```python
from build123d import *

# Parameters (mm, degrees)
SKETCH1_W           = 40.64
SKETCH1_H           = 32
BOSS_EXTRUDE1_DEPTH = 4
SKETCH2_R           = 8
BOSS_EXTRUDE2_DEPTH = 3.6
SKETCH3_W           = 3.3
SKETCH3_H           = 32
BOSS_EXTRUDE3_DEPTH = 3.6
FILLET1_R           = 0.5


with BuildPart() as part:
    # Sketch1 → Boss-Extrude1 (new body)
    with BuildSketch(Plane(origin=(0, 0, 0), x_dir=(1, 0, 0), z_dir=(0, 1, 0))):
        Rectangle(SKETCH1_W, SKETCH1_H)
    extrude(amount=BOSS_EXTRUDE1_DEPTH)

    # Sketch2 → Boss-Extrude2 (add)
    with BuildSketch(Plane(origin=(0, 4, 0), x_dir=(1, 0, 0), z_dir=(0, 1, 0))):
        with Locations(Location((0, 0, 0), (0, 0, 270))):
            Circle(SKETCH2_R)
    extrude(amount=BOSS_EXTRUDE2_DEPTH)

    # Sketch3 → Boss-Extrude3 (add)
    with BuildSketch(Plane(origin=(0, 4, 0), x_dir=(1, 0, 0), z_dir=(0, 1, 0))):
        with Locations((-18.67, 0)):
            Rectangle(SKETCH3_W, SKETCH3_H)
    boss_extrude3 = extrude(amount=BOSS_EXTRUDE3_DEPTH)

    # Mirror1: Boss-Extrude3 across plane
    add(boss_extrude3.mirror(Plane(origin=(0, 0, 0), x_dir=(0, 0, 1), z_dir=(1, 0, 0))))

    # Fillet1
    fillet1_edges = [part.edges().sort_by_distance(p)[0] for p in [
        (-17.02, 5.8, 16),
        (-17.02, 5.8, -16),
        (17.02, 5.8, 16),
        (17.02, 5.8, -16),
        (20.32, 3.8, 16),
        (-20.32, 3.8, 16),
        (-20.32, 3.8, -16),
        (20.32, 3.8, -16),
    ]]
    fillet(fillet1_edges, radius=FILLET1_R)


solid = part.part
```
Geometry: final body of the model. Coordinates: model frame, mm. A direction names the side the tool comes from. Coordinates: 2 decimals unless noted, no trailing zeros. Order: outer loops, then holes, each group sorted by start corner. A loop starts at its lowest first (then second) coordinate and runs counter-clockwise, first axis right, second up. Notation, with made-up numbers: M 11,26.25 L 16,26.25 A31 ccw 16,65.25 Z; hole C -23,-23 d4. An arc over 180 degrees is marked long. Answer as CSV lines item,"result".
Q1. Draft query along X for faces 1 (the flat face through (-19, 7.6, 0)), 2 (the flat face through (20.32, 4, 0)), 3 (the flat face through (-4.1, 4, -7.3)), 4 (the flat face through (-17.02, 6, 0)). Return one class per face: pulls with the +X half, pulls with the -X half, needs draft (parallel to the pull), parting line crosses it, or undercut.
Answers:
face 1,"needs draft"
face 2,"pulls with the +X half"
face 3,"undercut"
face 4,"undercut"
Q2. Set-up query: faces 5 (the flat face through (-20.32, 4, 0)), 6 (the flat face through (17.02, 6, 0)), 7 (the cylindrical face through (-7.81, 5.77, -1.73)). Return all of +Z, -Z, +X, -X, +Y, -Y with unobstructed straight access to the full face (end or side cutting, diameter ignored); none if empty.
Answers:
face 5,"+Z, -Z, -X, +Y, -Y"
face 6,"+Z, -Z, +Y"
face 7,"+Y"
Q3. Section B-B on z = 10.5. Return the cut outline in (x, y), and give its area (3 significant figures).
Answers:
outline,"M -20.32,0 L 20.32,0 L 20.32,7.6 L 17.02,7.6 L 17.02,4 L -17.02,4 L -17.02,7.6 L -20.32,7.6 Z"
area,"186 mm^2"
Q4. Section C-C on x = 0. Return the cut outline in (y, z), and give its area (3 significant figures).
Answers:
outline,"M 0,-16 L 4,-16 L 4,-8 L 7.6,-8 L 7.6,8 L 4,8 L 4,16 L 0,16 Z"
area,"186 mm^2"
Q5. Line query: probe 1 along X at (y, z) = (7, 9); probe 2 along X at (y, z) = (5, -5) (3 decimals); probe 3 along Y at (x, z) = (-10.5, -11). Output: solid intervals per line, ascending. Write a range as [from, to].
Answers:
probe 1,"x = [-20.32, -17.02], [17.02, 20.32]"
probe 2,"x = [-20.32, -17.02], [-6.245, 6.245], [17.02, 20.32]"
probe 3,"y = [0, 4]"
Q6. Section A-A on y = 6.25. Return the cut outline in (x, z), and give its area (3 significant figures).
Answers:
outline,"M -20.32,-15.5 A0.5 ccw -19.82,-16 L -17.52,-16 A0.5 ccw -17.02,-15.5 L -17.02,15.5 A0.5 ccw -17.52,16 L -19.82,16 A0.5 ccw -20.32,15.5 Z; C 0,0 d16; M 17.02,-15.5 A0.5 ccw 17.52,-16 L 19.82,-16 A0.5 ccw 20.32,-15.5 L 20.32,15.5 A0.5 ccw 19.82,16 L 17.52,16 A0.5 ccw 17.02,15.5 Z"
area,"412 mm^2"
Q7. First-contact query: P1, Ø1.5, axis at x = 9.5, y = 6, coming from the -Z side. Flat tip, straight axial feed; report the tip coordinate or a pass-through.
Answers:
P1,"passes through"
Q8. Section D-D on z = 0. Return the cut outline in (x, y).
Answers:
outline,"M -20.32,0 L 20.32,0 L 20.32,7.6 L 17.02,7.6 L 17.02,4 L 8,4 L 8,7.6 L -8,7.6 L -8,4 L -17.02,4 L -17.02,7.6 L -20.32,7.6 Z"
